Design review of the part built by this model. Coordinates are the model's own, in mm. A direction names the side the tool comes from. Give positions to 0.01 mm unless a question says otherwise; leave off trailing zeros. Loops run counter-clockwise (first coordinate to the right, second up) from the corner with the lowest first, then second, coordinate; pieces in that order, holes last. Notation, with made-up numbers: (67, -20) -> (77, -20) arc R11 ccw to (77, -5) -> close; hole circle Ø3 at (0.5, -32). An arc over 180 degrees is marked (long way). Answer as CSV lines item,"result".
from build123d import *

# Parameters (mm, degrees)
SKETCH_1_R          = 1.6
EXTRUDE_1_DEPTH     = 3
SKETCH_4_W          = 10
SKETCH_4_H          = 3
EXTRUDE_2_DEPTH     = 3
SKETCH_5_R          = 1.1
CUT_EXTRUDE_1_DEPTH = 200.90049168
FILLET_1_R          = 20
FILLET_2_R          = 9
SKETCH_6_W          = 55
SKETCH_6_H          = 21.983396943
CUT_EXTRUDE_2_DEPTH = 200.90049168
FILLET_3_R          = 6
FILLET_4_R          = 3
FILLET_5_R          = 20
CHAMFER_1_SIZE      = 8
CHAMFER_3_SIZE      = 20
CHAMFER_3_SIZE2     = 9.326153163


with BuildPart() as part:
    # 草图1 → 凸台-拉伸1 (new body)
    with BuildSketch(Plane.XY):
        Polygon((-47.5, -22.5), (-47.5, 22.5), (32.5, 78.516603057), (182.5, 78.516603057), (182.5, 58.516603057), (47.5, 58.516603057), (47.5, -9.483396943), (182.5, -9.483396943), (182.5, -29.483396943), (-28.313274587, -29.483396943), align=None)
        with Locations((-37.5, 7.5)):
            Circle(SKETCH_1_R, mode=Mode.SUBTRACT)
        with Locations((-37.5, -12.5)):
            Circle(SKETCH_1_R, mode=Mode.SUBTRACT)
        with Locations((37.5, 7.5)):
            Circle(SKETCH_1_R, mode=Mode.SUBTRACT)
        with Locations((37.5, -12.5)):
            Circle(SKETCH_1_R, mode=Mode.SUBTRACT)
    extrude(amount=EXTRUDE_1_DEPTH)

    # 草图4 → 凸台-拉伸2 (add)
    with BuildSketch(Plane.XY.offset(3)):
        with Locations((132.5, 80.016603057)):
            Rectangle(SKETCH_4_W, SKETCH_4_H)
        with Locations((172.5, 80.016603057)):
            Rectangle(SKETCH_4_W, SKETCH_4_H)
        with Locations((132.5, -7.983396943)):
            Rectangle(SKETCH_4_W, SKETCH_4_H)
        with Locations((172.5, -7.983396943)):
            Rectangle(SKETCH_4_W, SKETCH_4_H)
    extrude(amount=-EXTRUDE_2_DEPTH)

    # 草图5 → 切除-拉伸1 (cut, through all)
    with BuildSketch(Plane.XY.offset(3)):
        with Locations((77, -13.983396943)):
            Circle(SKETCH_5_R)
        with Locations((118, -13.983396943)):
            Circle(SKETCH_5_R)
        with Locations((97.5, -27.833396943)):
            Circle(SKETCH_5_R)
        with Locations((77, 63.016603057)):
            Circle(SKETCH_5_R)
        with Locations((118, 63.016603057)):
            Circle(SKETCH_5_R)
        with Locations((97.5, 76.866603057)):
            Circle(SKETCH_5_R)
        Polygon((150.9, 78.516603057), (154.1, 78.516603057), (154.1, 74.516603057), (156, 74.516603057), (156, 71.516603057), (154.1, 71.516603057), (154.1, 69.516603057), (150.9, 69.516603057), (150.9, 71.516603057), (149, 71.516603057), (149, 74.516603057), (150.9, 74.516603057), align=None)
        Polygon((150.9, -9.483396943), (154.1, -9.483396943), (154.1, -13.483396943), (156, -13.483396943), (156, -16.483396943), (154.1, -16.483396943), (154.1, -18.483396943), (150.9, -18.483396943), (150.9, -16.483396943), (149, -16.483396943), (149, -13.483396943), (150.9, -13.483396943), align=None)
    extrude(amount=-CUT_EXTRUDE_1_DEPTH, mode=Mode.SUBTRACT)

    # 圆角1
    fillet_1_edges = [part.edges().sort_by_distance(p)[0] for p in [
        (47.5, 58.516603057, 1.5),
    ]]
    fillet(fillet_1_edges, radius=FILLET_1_R)

    # 圆角2
    fillet_2_edges = [part.edges().sort_by_distance(p)[0] for p in [
        (47.5, -9.483396943, 1.5),
    ]]
    fillet(fillet_2_edges, radius=FILLET_2_R)

    # 草图6 → 切除-拉伸2 (cut, through all)
    with BuildSketch(Plane.XY.offset(3)):
        with BuildLine():
            Line((-22.5, 25.35589339), (36.283585467, 66.516603057))
            Line((36.283585467, 66.516603057), (46.5, 66.516603057))
            ThreePointArc((46.5, 66.516603057), (36.195048315, 54.169078899), (32.5, 38.516603057))
            Line((32.5, 38.516603057), (32.5, 17.5))
            Line((32.5, 17.5), (-22.5, 17.5))
            Line((-22.5, 17.5), (-22.5, 25.35589339))
        make_face()
        with Locations((0, -8.491698472)):
            Rectangle(SKETCH_6_W, SKETCH_6_H)
    extrude(amount=-CUT_EXTRUDE_2_DEPTH, mode=Mode.SUBTRACT)

    # 圆角3
    fillet_3_edges = [part.edges().sort_by_distance(p)[0] for p in [
        (27.5, 2.5, 1.5),
        (27.5, -19.483396943, 1.5),
        (-27.5, -19.483396943, 1.5),
        (-27.5, 2.5, 1.5),
    ]]
    fillet(fillet_3_edges, radius=FILLET_3_R)

    # 圆角4
    fillet_4_edges = [part.edges().sort_by_distance(p)[0] for p in [
        (-22.5, 17.5, 1.5),
        (-22.5, 25.35589339, 1.5),
        (36.283585467, 66.516603057, 1.5),
        (46.5, 66.516603057, 1.5),
        (32.5, 17.5, 1.5),
    ]]
    fillet(fillet_4_edges, radius=FILLET_4_R)

    # 圆角5
    fillet_5_edges = [part.edges().sort_by_distance(p)[0] for p in [
        (32.5, 78.516603057, 1.5),
    ]]
    fillet(fillet_5_edges, radius=FILLET_5_R)

    # 倒角1
    chamfer_1_edges = [part.edges().sort_by_distance(p)[0] for p in [
        (182.5, 58.516603057, 1.5),
    ]]
    chamfer(chamfer_1_edges, length=CHAMFER_1_SIZE)

    # 倒角3
    chamfer_3_edges = [part.edges().sort_by_distance(p)[0] for p in [
        (182.5, -29.483396943, 1.5),
    ]]
    chamfer_3_side = [part.faces().sort_by_distance(p)[0] for p in [
        (77.093362706, -29.483396943, 1.5),
    ]]
    chamfer(chamfer_3_edges, length=CHAMFER_3_SIZE, length2=CHAMFER_3_SIZE2, reference=chamfer_3_side[0])


solid = part.part
Q1. We need section C-C, the plane y = 49.5. State the section outline as (x, z) points.
Filled sheet:
outline,"(-8.94, 0) -> (11.98, 0) -> (11.98, 3) -> (-8.94, 3) -> close; (34.27, 0) -> (50.79, 0) -> (50.79, 3) -> (34.27, 3) -> close"
Q2. We need section B-B, the plane z = 1.25. State how many separate pieces and enclosed holes the cut face has, and give its area (3 significant figures).
Filled sheet:
separate pieces,"1"
enclosed holes,"12"
area,"10,500 mm^2"
Q3. For faces 1 (the flat face through (-10.61, 48.33, 1.48)), 2 (the flat face through (178.444, 62.461, 1.479)), 3 (the cylindrical face through (25.79, -17.68, 1.48)), list the 3-axis set-ups (+Z, -Z, +X, -X, +Y, -Y) from which the entire face can be reached by the end or side of a thin tool; tool diameter is ignored.
Filled sheet:
face 1,"+Z, -Z, -X, +Y"
face 2,"+Z, -Z, +X"
face 3,"+Z, -Z"
Q4. We need section A-A, the plane y = 34. State the section outline as (x, z) points, and give its area (3 significant figures).
Filled sheet:
outline,"(-31.08, 0) -> (-10.15, 0) -> (-10.15, 3) -> (-31.08, 3) -> close; (32.5, 0) -> (47.5, 0) -> (47.5, 3) -> (32.5, 3) -> close"
area,"108 mm^2"
Q5. To check wall thickness, follow probe 1 along X at (y, z) = (-10.5, 0.1); probe 2 along Y at (x, z) = (37.5, 1.5); probe 3 along Y at (x, z) = (97.5, 1.95). State the ranges of each line that lie inside material, in increasing order. Write a range as from..to.
Filled sheet:
probe 1,"x = -47.5..-27.5, 27.5..150.9, 154.1..182.5"
probe 2,"y = -29.48..-14.1, -10.9..5.9, 9.1..56.54, 66.52..78.47"
probe 3,"y = -29.48..-28.93, -26.73..-9.48, 58.52..75.77, 77.97..78.52"
Q6. Clearance check with flat-ended pins moving along their axes: pin 1 Ø1.5 at (x, z) = (143, 1) entering from +Y; pin 2 Ø0.9 at (y, z) = (22.5, 2) entering from +X. State where each tip first meets the part, or that it passes through.
Filled sheet:
pin 1,"stops at y = 78.52"
pin 2,"stops at x = 47.5"
Q7. The part is to be moulded in two halves that separate along X. For faces 4 (the flat face through (44, 27, 0)), 5 (the flat face through (172.64, -24.755, 1.479)), 6 (the flat face through (6.7, 45.8, 1.5)), say which applies: pulls with the +X half, pulls with the -X half, needs draft (parallel to the pull), parting line crosses it, or undercut.
Filled sheet:
face 4,"needs draft"
face 5,"pulls with the +X half"
face 6,"undercut"
